Can you work these out from the model? Positions are in its coordinate system, mm. A direction names the side the tool comes from. Round coordinates to 2 decimals unless told otherwise and drop trailing zeros. Write each loop counter-clockwise with the first axis right and the second up, starting at its lowest first coordinate (ties: lowest second). Pieces come first, ordered by that corner, then holes. Notation, with made-up numbers: M 67.5,40.5 L 123.5,40.5 A32 cw 123.5,77.5 Z; hole C 17,21 d4. An arc over 180 degrees is marked long. Answer as a JSON object with one key per item and string values. Group by question number.
1) Suppose I cut it at B-B, the plane x = 24. Write out the boundary of the cut face in (y, z).
2) Please list where these lines run through material, in increasing order: L1, parallel to X at y = 44, z = 0; L2, parallel to X at y = 51.25, z = 0; L3, parallel to Z at x = -21, y = 49. Write a range as [from, to].
3) Suppose I cut it at A-A, the plane z = 0. Write out the boundary of the cut face in (x, y), and give its area (3 significant figures).
4) I'm going to push flat-ended pins straight in: pin 1 Ø4 at (x, z) = (-19.84, 0) entering from -Y; pin 2 Ø1 at (x, y) = (-20, 17) entering from -Z; pin 3 Ø1 at (y, z) = (10, -6.5) entering from +X; pin 4 Ø6 at (y, z) = (7, -3.5) entering from -X. Where does each tip first touch, or does it pass through?
5) Suppose I cut it at D-D, the plane x = -21. Write out the boundary of the cut face in (y, z), and give its area (3 significant figures).
6) If we mould it in two halves opening along Z, with no side actions, what happens to faces 1 (the cylindrical face through (-28.977, 29.58, -1.162)), 2 (the flat face through (-16, 60, 0)), 3 (the flat face through (20, 20, 8))? For each: +Z half, -Z half, draft (parallel to the pull), parting line (faces both ways), or undercut.
7) Suppose I cut it at C-C, the plane y = 5. Write out the boundary of the cut face in (x, z).
8) On a 3-axis mill with a long thin cutter (end or side, diameter ignored), from which of +Z, -Z, +X, -X, +Y, -Y can I reach the whole of each face in a straight line? I mean faces 4 (the cylindrical face through (-22.94, 50.14, 1.62)), 5 (the flat face through (20, 20, -8)), 6 (the flat face through (3.946, 51.465, 0.406)). Say none if no direction works.
from build123d import *

# Parameters (mm, degrees)
SKETCH3_R           = 29
BOSS_EXTRUDE1_DEPTH = 60
CUT_EXTRUDE1_DEPTH  = 30
SKETCH8_R           = 3.5
CUT_EXTRUDE2_DEPTH  = 20
SKETCH15_W          = 16
SKETCH15_H          = 16
CUT_EXTRUDE4_DEPTH  = 61


with BuildPart() as part:
    # Sketch3 → Boss-Extrude1 (new body)
    with BuildSketch(Plane(origin=(0, 0, 0), x_dir=(1, 0, 0), z_dir=(0, 1, 0))):
        with Locations(Location((0, 0, 0), (0, 0, 270))):
            Circle(SKETCH3_R)
    extrude(amount=BOSS_EXTRUDE1_DEPTH)

    # Sketch6 → Cut-Extrude1 (cut, symmetric)
    with BuildSketch(Plane.XY):
        Polygon((-10.837168574, 60), (29, 37), (29, 60), align=None)
    extrude(amount=CUT_EXTRUDE1_DEPTH, both=True, mode=Mode.SUBTRACT)

    # Sketch8 → Cut-Extrude2 (cut)
    with BuildSketch(Plane(origin=(0, 60, 0), x_dir=(1, 0, 0), z_dir=(0, 1, 0))):
        with Locations(Location((-19.837168574, 0, 0), (0, 0, 270))):
            Circle(SKETCH8_R)
    extrude(amount=-CUT_EXTRUDE2_DEPTH, mode=Mode.SUBTRACT)

    # Sketch15 → Cut-Extrude4 (cut, along a direction that is not the sketch's normal)
    with BuildSketch(Plane(origin=(23.27146997, 40.307368355, 0), x_dir=(0.8660254037844416, -0.49999999999999484, 0), z_dir=(0.49999999999999484, 0.8660254037844416, 0))):
        with Locations((-1.38526329, 0)):
            Rectangle(SKETCH15_W, SKETCH15_H)
    extrude(amount=-CUT_EXTRUDE4_DEPTH, dir=(0, 1, 0), mode=Mode.SUBTRACT)


solid = part.part
Results:
{
 "1": {"outline": "M 0,-16.28 L 39.89,-16.28 L 39.89,-8 L 0,-8 Z; M 0,8 L 39.89,8 L 39.89,16.28 L 0,16.28 Z"},
 "2": {"L1": "[-29, -23.34], [-16.34, 15.14]", "L2": "[-29, -23.34], [-16.34, 4.32]", "L3": "[-20, -3.3], [3.3, 20]"},
 "3": {"outline": "M -29,0 L 15.14,0 L 15.14,45 L -10.84,60 L -16.34,60 L -16.34,40 L -23.34,40 L -23.34,60 L -29,60 Z", "area": "2,310 mm^2"},
 "4": {"pin 1": "y = 0", "pin 2": "z = -21.47", "pin 3": "x = 15.14", "pin 4": "x = -29"},
 "5": {"outline": "M 0,-20 L 60,-20 L 60,-3.3 L 40,-3.3 L 40,3.3 L 60,3.3 L 60,20 L 0,20 Z", "area": "2,270 mm^2"},
 "6": {"face 1": "parting line", "face 2": "draft", "face 3": "undercut"},
 "7": {"outline": "M 15.14,-8 L 15.14,8 L 27.87,8 A29 ccw long 27.87,-8 Z"},
 "8": {"face 4": "+Y", "face 5": "+X, +Y, -Y", "face 6": "+Z, -Z, +X, +Y"}
}
